Part print with two shaded views. Sizes in mm from the minimum x, y, z corner. Coordinates: 2 decimals unless noted, no trailing zeros. Loops run counter-clockwise (first coordinate to the right, second up) from the corner with the lowest first, then second, coordinate; pieces in that order, holes last. Notation, with made-up numbers: (-12.5, 88.25) -> (11.5, 88.25) arc R12 cw to (11.5, 105.25) -> close; hole circle Ø7 at (-22.75, 58). An arc over 180 degrees is marked (long way). One line per item, written item: value. Start each with the question number.
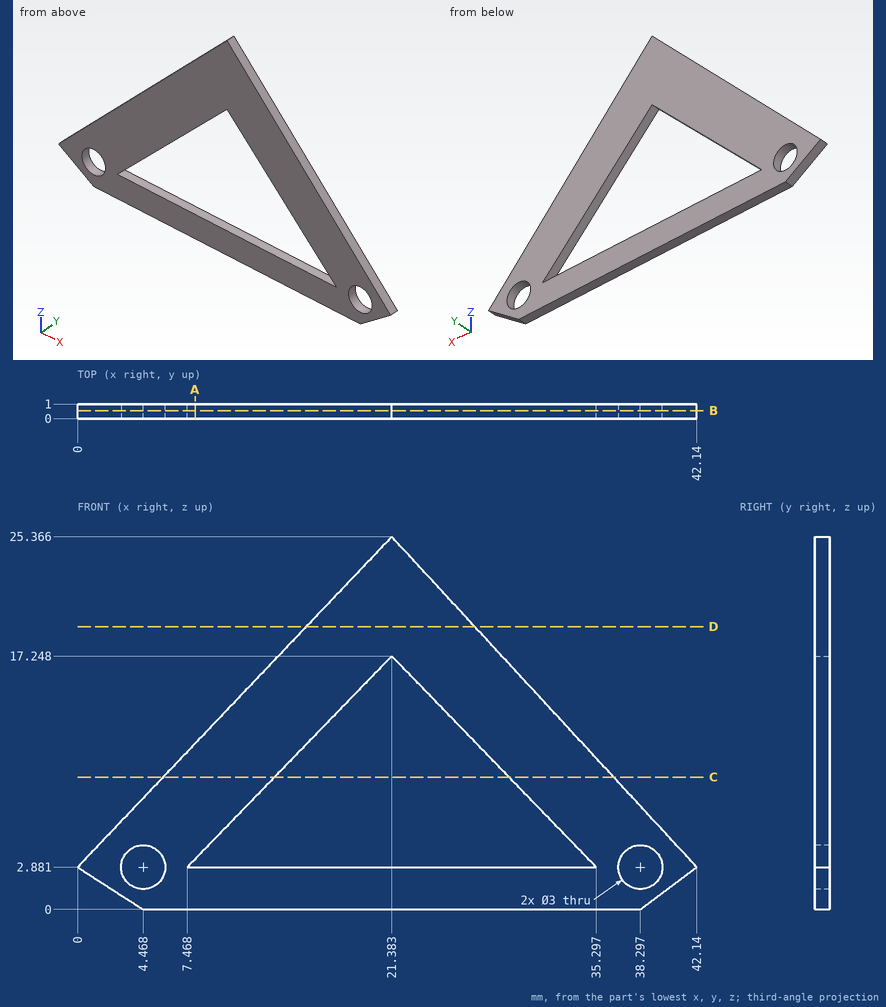
Item 1: Band-saw the part on C-C, the plane z = 9. List the corners of the cut face in (x, y) (1 decimal).
Item 2: Band-saw the part on D-D, the plane z = 19.25. List the corners of the cut face in (x, y).
Item 3: Probe probe 1 along X at (y, z) = (0.95, 6.5) (1 decimal); probe 2 along Z at (x, y) = (14, 0.2) (1 decimal); probe 3 along Z at (x, y) = (11.5, 0.5) (1 decimal). List the from-to ranges inside material, lowest first.
Item 4: Band-saw the part on B-B, the plane y = 0.55. List the corners of the cut face in (x, z), and give its area (3 significant figures).
Item 5: Band-saw the part on A-A, the plane x = 8. List the corners of the cut face in (y, z).
Worked out:
1. outline: (5.8, 0) -> (13.4, 0) -> (13.4, 1) -> (5.8, 1) -> close; (29.4, 0) -> (36.5, 0) -> (36.5, 1) -> (29.4, 1) -> close
2. outline: (15.57, 0) -> (27.03, 0) -> (27.03, 1) -> (15.57, 1) -> close
3. probe 1: x = 3.4 to 11, 31.8 to 38.8
3. probe 2: z = 0 to 2.9, 9.6 to 17.6
3. probe 3: z = 0 to 2.9, 7 to 15
4. outline: (0, 2.88) -> (4.47, 0) -> (38.3, 0) -> (42.14, 2.88) -> (21.38, 25.37) -> close; hole circle Ø3 at (4.47, 2.88); hole (7.47, 2.88) -> (35.3, 2.88) -> (21.38, 17.25) -> close; hole circle Ø3 at (38.3, 2.88)
4. area: 369 mm²
5. outline: (0, 0) -> (1, 0) -> (1, 2.88) -> (0, 2.88) -> close; (0, 3.43) -> (1, 3.43) -> (1, 11.29) -> (0, 11.29) -> close
